The model under review builds one solid part; all positions refer to its coordinate system, in mm. Face numbers are marked on the shaded views. A direction names the side the tool comes from. Give positions to 0.01 mm unless a question says otherwise; leave off trailing zeros. Write each loop counter-clockwise with the first axis right and the second up, starting at its lowest first coordinate (ties: lowest second). Pieces come first, ordered by that corner, then holes. Notation, with made-up numbers: (37.25, -32) - (71.25, -32) arc R3 cw to (71.25, -27) - close; hole circle Ø2 at (6.25, -37). An arc over 180 degrees is marked (long way). Write item = value, one per line.
```python
from build123d import *

# Parameters (mm, degrees)
SKETCH_1_W          = 117
SKETCH_1_H          = 117
SKETCH_1_R          = 39
EXTRUDE_1_DEPTH     = 40
CUT_EXTRUDE_1_REACH = 119
SKETCH_2_W          = 36
SKETCH_2_H          = 40
SKETCH_7_W          = 9.65
SKETCH_7_H          = 20.5
CUT_EXTRUDE_4_DEPTH = 40
CUT_EXTRUDE_5_DEPTH = 15
SKETCH_9_W          = 31
SKETCH_9_H          = 20.5
CUT_EXTRUDE_6_DEPTH = 35


with BuildPart() as part:
    # 草圖1 → 填料-伸長1 (new body)
    with BuildSketch(Plane.XY):
        with Locations((4.648877503, -26.451389471)):
            Rectangle(SKETCH_1_W, SKETCH_1_H)
        with Locations((4.648877503, -26.451389471)):
            Circle(SKETCH_1_R, mode=Mode.SUBTRACT)
    extrude(amount=EXTRUDE_1_DEPTH)

    # 草圖2 → 除料-伸長1 (cut, up to next)
    with BuildSketch(Plane.XZ.offset(84.951389471), mode=Mode.PRIVATE) as cut_extrude_1_sk1:
        with Locations((4.648877503, 20)):
            Rectangle(SKETCH_2_W, SKETCH_2_H)
    cut_extrude_1_tool1 = extrude(cut_extrude_1_sk1.sketch, amount=-CUT_EXTRUDE_1_REACH, mode=Mode.PRIVATE) & part.part
    add(cut_extrude_1_tool1.solids().sort_by_distance((4.648878, -84.951389, 20))[0], mode=Mode.SUBTRACT)

    # 草圖7 → 除料-伸長4 (cut)
    with BuildSketch(Plane.XY.offset(40)):
        with Locations((27.473877503, -69.701389471)):
            Rectangle(SKETCH_7_W, SKETCH_7_H)
    extrude(amount=-CUT_EXTRUDE_4_DEPTH, mode=Mode.SUBTRACT)

    # 草圖8 → 除料-伸長5 (cut)
    with BuildSketch(Plane(origin=(-13.351122497, 0, 0), x_dir=(0, 0, -1), z_dir=(1, 0, 0))):
        with BuildLine():
            Line((-40, -66.451389471), (-40, -73.451389471))
            Line((-40, -73.451389471), (-35, -73.451389471))
            ThreePointArc((-35, -73.451389471), (-38.5, -69.951389471), (-35, -66.451389471))
            Line((-35, -66.451389471), (-40, -66.451389471))
        make_face()
        with BuildLine():
            ThreePointArc((-35, -66.451389471), (-38.5, -69.951389471), (-35, -73.451389471))
            Line((-35, -73.451389471), (-35, -66.451389471))
        make_face()
        with BuildLine():
            Line((-35, -66.451389471), (-35, -73.451389471))
            ThreePointArc((-35, -73.451389471), (-32.525126266, -72.426263205), (-31.5, -69.951389471))
            ThreePointArc((-31.5, -69.951389471), (-32.525126266, -67.476515737), (-35, -66.451389471))
        make_face()
    extrude(amount=-CUT_EXTRUDE_5_DEPTH, mode=Mode.SUBTRACT)

    # 草圖9 → 除料-伸長6 (cut)
    with BuildSketch(Plane.XY.offset(40)):
        with Locations((47.798877503, -69.701389471)):
            Rectangle(SKETCH_9_W, SKETCH_9_H)
    extrude(amount=-CUT_EXTRUDE_6_DEPTH, mode=Mode.SUBTRACT)


solid = part.part
```
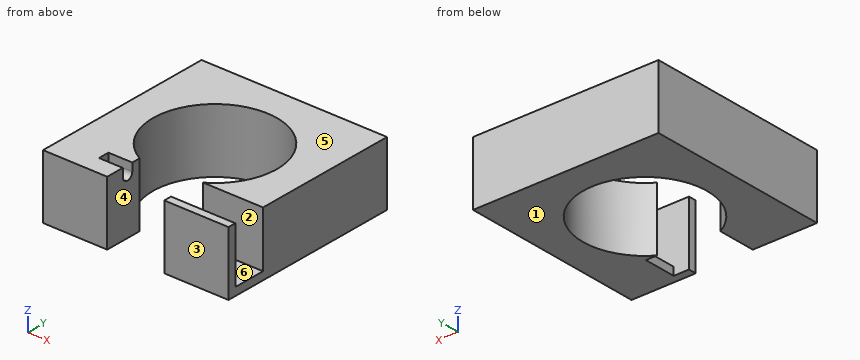
1. Take a section at D-D on x = 30.5. Give the boundary of the cut face in (y, z), and give its area (3 significant figures).
Findings below:
outline = (-84.95, 0) - (-79.95, 0) - (-79.95, 40) - (-84.95, 40) - close; (-59.45, 0) - (-55.65, 0) - (-55.65, 40) - (-59.45, 40) - close; (2.75, 0) - (32.05, 0) - (32.05, 40) - (2.75, 40) - close
area = 1,520 mm²
2. Machinability: for the marked faces 4, 5 and 6, which of the approach directions +Z, -Z, +X, -X, +Y, -Y give a long, thin tool a straight path to every point of the face, cutting with its end or side? Answer none if there is none.
Findings below:
face_4 = +Z, -Z, -Y
face_5 = +Z, +X, -X, +Y, -Y
face_6 = +Z, +X
3. For line 1 (Y direction, x = 48, z = 28); line 2 (Y direction, x = -16.5, z = 34); line 3 (Z direction, x = 45.5, y = -63.5), list the stretches that pass through material, from the lowest coordinate up. Write a range as from..to.
Findings below:
line_1 = -84.95..-79.95, -59.45..32.05
line_2 = -84.95..-73.31, -66.6..-59.22, 6.32..32.05
line_3 = 0..5
4. Take a section at A-A on z = 27. Give the boundary of the cut face in (x, y), and give its area (3 significant figures).
Findings below:
outline = (-53.85, -84.95) - (-13.35, -84.95) - (-13.35, -61.05) arc R39 cw (long way) to (25.43, -59.45) - (63.15, -59.45) - (63.15, 32.05) - (-53.85, 32.05) - close; (22.65, -84.95) - (63.15, -84.95) - (63.15, -79.95) - (22.65, -79.95) - close
area = 7,330 mm²
5. Insertion check: P1, Ø12, axis at x = -42, y = -12.5, coming from the -Z side; P2, Ø7, axis at y = -74, z = 14.5, coming from the +X side; P3, Ø5, axis at x = -2, z = 16.5, coming from the -Y side. Each pin has a flat end and moves straight along its axis. Give the tip position at first contact, or say it passes through.
Findings below:
P1 = 0
P2 = -13.35
P3 = 11.46
6. Draft analysis for pull direction Y (two halves, no side actions). For the marked faces 1, 2 and 3, state which applies: +Y half, -Y half, draft (parallel to the pull), parting line (faces both ways), or undercut.
Findings below:
face_1 = draft
face_2 = undercut
face_3 = -Y half
7. Take a section at B-B on x = -16.5. Give the boundary of the cut face in (y, z).
Findings below:
outline = (-84.95, 0) - (-59.22, 0) - (-59.22, 40) - (-66.45, 40) - (-66.45, 35) arc R3.5 cw to (-73.45, 35) - (-73.45, 40) - (-84.95, 40) - close; (6.32, 0) - (32.05, 0) - (32.05, 40) - (6.32, 40) - close
8. Take a section at C-C on y = -24. Give the boundary of the cut face in (x, z).
Findings below:
outline = (-53.85, 0) - (-34.27, 0) - (-34.27, 40) - (-53.85, 40) - close; (43.57, 0) - (63.15, 0) - (63.15, 40) - (43.57, 40) - close
